The listing builds one solid part. Answer for the finished solid, in the listing's coordinates (mm). A direction names the side the tool comes from. Round coordinates to 2 decimals unless told otherwise and drop trailing zeros. Order: outer loops, then holes, each group sorted by start corner. A loop starts at its lowest first (then second) coordinate and runs counter-clockwise, first axis right, second up. Notation, with made-up numbers: M 6,-17 L 22,-17 A27 cw 22,15 Z; hole C 59.5,4 d6. An arc over 180 degrees is marked long. Write item = value, one per line. Start each with the question number.
(1) For a pull along Z with two mould halves and no side action, classify faces 1 (the face through (145, 0, -31)), 2 (the face through (89.865, -1.521, -6.162)), 3 (the face through (243.649, 0, -55)), 4 (the face through (135, 0, -60)) as released by +Z, released by -Z, zero draft, split by the parting line, or undercut.
(2) A cutting plane is placed at A-A, the plane y = 1.8. Determine the outline of the cut face in (x, z).
(3) This flat-tipped pin is pushed along its axis until it touches: pin 1 (7 mm diameter, centred on x = 90, z = -6, fed in from +Y). Where does it stop, or does it pass through?
(4) A cutting plane is placed at B-B, the plane x = 217.5. Determine the outline of the cut face in (y, z), and give its area (3 significant figures).
(5) A cutting plane is placed at C-C, the plane x = 188. Determine the outline of the cut face in (y, z), and give its area (3 significant figures).
(6) Straight lines are drawn through the part: probe 1 along Z at (x, y) = (39.5, 2.6); probe 2 along Z at (x, y) = (138, 2.6); probe 3 along Z at (x, y) = (225, 1.05). For each, find the intervals that lie inside material, in ascending order. Write a range as from..to.
(7) Which of the six approach directions +Z, -Z, +X, -X, +Y, -Y give full straight-line access (tool end or side, diameter ignored) to faces 5 (the face through (112, 3, -36)), 6 (the face through (145.35, 1.48, -31.85)), 7 (the face through (30, 0, -5)), 8 (the face through (89, 0, -8)), 9 (the face through (35, 0, -10))?
from build123d import *

# Parameters (mm, degrees)
F1_DEPTH = 3
F3_DEPTH = 3


with BuildPart() as f1:
    # F0 (on Front) → F1 (new body)
    with BuildSketch(Plane.XZ):
        Polygon((146.8245836552, -25), (50, 0), (30, 0), (30, -10), (40, -10), (40, -13), (30, -13), (30, -60), (243.6491673104, -60), (243.6491673104, -50), align=None)
        Polygon((126.4596669241, -23.8729833462), (145.8245836552, -28.8729833462), (165.1895003862, -33.8729833462), (164.4395003862, -36.7777208559), (125.7096669241, -26.7777208559), align=None, mode=Mode.SUBTRACT)
    extrude(amount=F1_DEPTH)

    # F2 (on face) + F0 (on Front) → F3 (join)
    with BuildSketch(Plane.XZ.offset(3)):
        Polygon((98.4122918276, -12.5), (79.0473750966, -7.5), (50, 0), (30, 0), (30, -10), (40, -10), (40, -13), (30, -13), (30, -60), (243.6491673104, -60), (243.6491673104, -50), (214.6017922138, -42.5), (195.2368754828, -37.5), align=None)
        Polygon((125.7096669241, -26.7777208559), (126.4596669241, -23.8729833462), (165.1895003862, -33.8729833462), (164.4395003862, -36.7777208559), align=None, mode=Mode.SUBTRACT)
        Polygon((165.1895003862, -33.8729833462), (126.4596669241, -23.8729833462), (125.7096669241, -26.7777208559), (164.4395003862, -36.7777208559), align=None)
        Polygon((80.0473750966, -3.6270166538), (79.0473750966, -7.5), (98.4122918276, -12.5), (99.4122918276, -8.6270166538), align=None)
    with BuildSketch(Plane.XZ):
        Polygon((146.8245836552, -25), (50, 0), (30, 0), (30, -10), (40, -10), (40, -13), (30, -13), (30, -60), (243.6491673104, -60), (243.6491673104, -50), align=None)
        Polygon((126.4596669241, -23.8729833462), (145.8245836552, -28.8729833462), (165.1895003862, -33.8729833462), (164.4395003862, -36.7777208559), (125.7096669241, -26.7777208559), align=None, mode=Mode.SUBTRACT)
    extrude(amount=-F3_DEPTH)


solid = f1.part
Reported:
q1.face_1 = undercut
q1.face_2 = released by +Z
q1.face_3 = zero draft
q1.face_4 = released by -Z
q2.outline = M 30,-60 L 243.65,-60 L 243.65,-50 L 50,0 L 30,0 L 30,-10 L 40,-10 L 40,-13 L 30,-13 Z; hole M 125.71,-26.78 L 164.44,-36.78 L 165.19,-33.87 L 126.46,-23.87 Z
q3.pin_1 = 0
q4.outline = M -3,-60 L 3,-60 L 3,-43.25 L -3,-43.25 Z
q4.area = 101 mm²
q5.outline = M -3,-60 L 3,-60 L 3,-35.63 L -3,-35.63 Z
q5.area = 146 mm²
q6.probe_1 = -60..-13, -10..0
q6.probe_2 = -60..-29.95, -26.85..-22.72
q6.probe_3 = -60..-45.18
q7.face_5 = +Z, -Z, +X, -X, +Y
q7.face_6 = +Y
q7.face_7 = +Z, -Z, -X, +Y, -Y
q7.face_8 = +Z, +X, +Y
q7.face_9 = -X, +Y, -Y
